Work out the finished part from the listing and answer in its coordinate system (mm). A direction names the side the tool comes from. Give positions to 0.01 mm unless a question says otherwise; leave off trailing zeros.
```python
from build123d import *

# Parameters (mm, degrees)
F0_W        = 50
F0_H        = 46.7033070608
F1_DEPTH    = 98.552
F1_TAPER    = -3
F2_T        = -2.54
F3_T1_DEPTH = 74.1036999946
F3_T3_DEPTH = 124.1528328785
F3_T5_DEPTH = 87.0957981099
F3_T7_DEPTH = 124.1528328785
F4_T1_DEPTH = 74.1036999946
F4_T3_DEPTH = 124.1528328785
F4_T5_DEPTH = 87.0957981099
F4_T7_DEPTH = 124.1528328785


# Not quite as in the source:
# - a fillet or chamfer that OpenCascade refuses, or shapes differently, is made with other operations: its cross-section is extruded or revolved along the edge and cut away or added


with BuildPart() as f1:
    # F0 (on Front) → F1 (new body)
    with BuildSketch(Plane.XZ):
        Rectangle(F0_W, F0_H)
    extrude(amount=F1_DEPTH, taper=F1_TAPER)

    # F2
    f2_openings = [f1.faces().sort_by_distance(p)[0] for p in [
        (0, -98.552, 0),
    ]]
    offset(amount=F2_T, openings=f2_openings)

    # F3: fillet of radius 5.08 on 4 edges, made by hand

    # F3_s2 → F3_t1 (cut)
    with BuildSketch(Plane.YZ.offset(-37.0518499973)):
        with BuildLine():
            ThreePointArc((-4.8141333423, 23.6039515681), (-1.3950981953, 22.027754776), (0, 18.5309135315))
            Line((0, 18.5309135315), (0, 23.3516535304))
            Line((0, 23.3516535304), (-4.8141333423, 23.6039515681))
        make_face()
    extrude(amount=F3_T1_DEPTH, mode=Mode.SUBTRACT)

    # F3_s4 → F3_t3 (cut)
    with BuildSketch(Plane(origin=(0.5298667006, 10.1104589396, -0.5298667006), x_dir=(0.9986295348, -0.0523359562, 0), z_dir=(-0.0522644277, -0.9972646886, 0.0522644277))):
        with BuildLine():
            ThreePointArc((-24.9657383689, 18.1852510398), (-23.4827569315, 21.7724306367), (-19.8996527546, 23.2652319837))
            Line((-19.8996527546, 23.2652319837), (-24.9657383689, 23.2513556581))
            Line((-24.9657383689, 23.2513556581), (-24.9657383689, 18.1852510398))
        make_face()
    extrude(amount=F3_T3_DEPTH, mode=Mode.SUBTRACT)

    # F3_s6 → F3_t5 (cut)
    with BuildSketch(Plane.YZ.offset(-43.547899055)):
        with BuildLine():
            ThreePointArc((-93.2061333423, 28.2363799944), (-96.9688412445, 26.8482437626), (-98.552, 23.1633419579))
            Line((-98.552, 23.1633419579), (-98.552, 28.5165449943))
            Line((-98.552, 28.5165449943), (-93.2061333423, 28.2363799944))
        make_face()
    extrude(amount=F3_T5_DEPTH, mode=Mode.SUBTRACT)

    # F3_s8 → F3_t7 (cut)
    with BuildSketch(Plane(origin=(-0.5298667006, 10.1104589396, -0.5298667006), x_dir=(0.9986295348, 0.0523359562, 0), z_dir=(0.0522644277, -0.9972646886, 0.0522644277))):
        with BuildLine():
            ThreePointArc((24.9657383689, 18.1852510398), (23.4827569315, 21.7724306367), (19.8996527546, 23.2652319837))
            Line((19.8996527546, 23.2652319837), (24.9657383689, 23.2513556581))
            Line((24.9657383689, 23.2513556581), (24.9657383689, 18.1852510398))
        make_face()
    extrude(amount=F3_T7_DEPTH, mode=Mode.SUBTRACT)

    # F4: fillet of radius 5.08 on 4 edges, made by hand

    # F4_s2 → F4_t1 (cut)
    with BuildSketch(Plane.YZ.offset(-37.0518499973)):
        with BuildLine():
            ThreePointArc((-4.8141333423, -23.6039515681), (-1.3950981953, -22.027754776), (0, -18.5309135315))
            Line((0, -18.5309135315), (0, -23.3516535304))
            Line((0, -23.3516535304), (-4.8141333423, -23.6039515681))
        make_face()
    extrude(amount=F4_T1_DEPTH, mode=Mode.SUBTRACT)

    # F4_s4 → F4_t3 (cut)
    with BuildSketch(Plane(origin=(-0.5298667006, 10.1104589396, 0.5298667006), x_dir=(0.9986295348, 0.0523359562, 0), z_dir=(0.0522644277, -0.9972646886, -0.0522644277))):
        with BuildLine():
            ThreePointArc((19.8996527546, -23.2652319837), (23.4827569315, -21.7724306367), (24.9657383689, -18.1852510398))
            Line((24.9657383689, -18.1852510398), (24.9657383689, -23.2513556581))
            Line((24.9657383689, -23.2513556581), (19.8996527546, -23.2652319837))
        make_face()
    extrude(amount=F4_T3_DEPTH, mode=Mode.SUBTRACT)

    # F4_s6 → F4_t5 (cut)
    with BuildSketch(Plane.YZ.offset(-43.547899055)):
        with BuildLine():
            ThreePointArc((-98.552, -23.1633419579), (-96.9688412445, -26.8482437626), (-93.2061333423, -28.2363799944))
            Line((-93.2061333423, -28.2363799944), (-98.552, -28.5165449943))
            Line((-98.552, -28.5165449943), (-98.552, -23.1633419579))
        make_face()
    extrude(amount=F4_T5_DEPTH, mode=Mode.SUBTRACT)

    # F4_s8 → F4_t7 (cut)
    with BuildSketch(Plane(origin=(0.5298667006, 10.1104589396, 0.5298667006), x_dir=(0.9986295348, -0.0523359562, 0), z_dir=(-0.0522644277, -0.9972646886, -0.0522644277))):
        with BuildLine():
            ThreePointArc((-24.9657383689, -18.1852510398), (-23.4827569315, -21.7724306367), (-19.8996527546, -23.2652319837))
            Line((-19.8996527546, -23.2652319837), (-24.9657383689, -23.2513556581))
            Line((-24.9657383689, -23.2513556581), (-24.9657383689, -18.1852510398))
        make_face()
    extrude(amount=F4_T7_DEPTH, mode=Mode.SUBTRACT)


solid = f1.part
```
1. Straight lines are drawn through the part: probe 1 along Z at (x, y) = (14, -69.5); probe 2 along X at (y, z) = (-88.5, 7); probe 3 along Y at (x, z) = (1.5, -12.5). For each, find the intervals that lie inside material, in ascending order.
Findings below:
probe 1: z = -26.99 to -24.45, 24.45 to 26.99
probe 2: x = -29.64 to -27.09, 27.09 to 29.64
probe 3: y = -2.54 to 0
2. The mould has two halves that part along Z. Classify faces 1 (the face through (-25.14, -51.22, 0.36)), 2 (the face through (26.016, -48.473, -24.446)), 3 (the face through (-1, 0, 0)): pulls with the +Z half, pulls with the -Z half, needs draft (parallel to the pull), parting line crosses it, or undercut.
Findings below:
face 1: undercut
face 2: pulls with the -Z half
face 3: needs draft
3. Given P1, Ø3, axis at x = -19.5, z = 14, coming from the -Y side; P2, Ø1.5, axis at y = -28.5, z = -16, coming from the -X side; P3, Ø6, axis at x = -19.5, y = -24, coming from the +Z side, each flat-ended and moving along its own axis, determine where each tip first touches the part or whether it passes through.
Findings below:
P1: stops at y = -2.54
P2: stops at x = -26.53
P3: stops at z = 24.77
4. Which of the six approach directions +Z, -Z, +X, -X, +Y, -Y give full straight-line access (tool end or side, diameter ignored) to faces 4 (the face through (-0.35, -1.432, -22.067)), 5 (the face through (0.39, -50.8, 23.47))?
Findings below:
face 4: -Z, +X, -X, +Y
face 5: -Y
